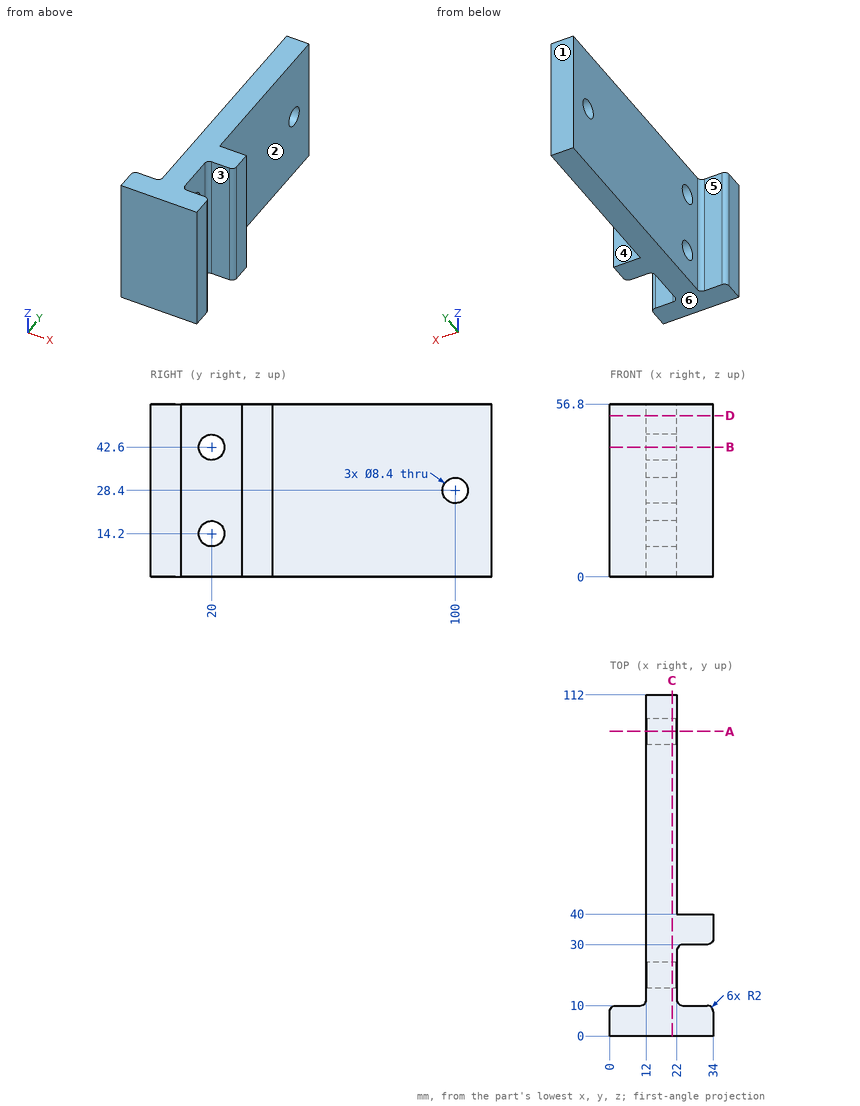
Study the drawing (mm; zero at the part's minimum x, y, z) and answer. A direction names the side the tool comes from. Round coordinates to 2 decimals unless told otherwise and drop trailing zeros. Loops run counter-clockwise (first coordinate to the right, second up) from the corner with the lowest first, then second, coordinate; pieces in that order, holes last. Notation, with made-up numbers: (-27, -36.5) -> (31, -36.5) arc R13 ccw to (31, -11.5) -> close; hole circle Ø10 at (-30, 75.5). An arc over 180 degrees is marked (long way). One line per item, written item: value.
1) For the marked faces 4, 5 and 6, determine the directions among +Z, -Z, +X, -X, +Y, -Y from which every point of the face is accessible in a straight line to the end or side of a thin tool.
Answer list:
face 4: +Z, -Z, +X, +Y
face 5: +Z, -Z, -X, +Y
face 6: -Z, +X, -X, +Y, -Y
2) The mould has two halves that part along Y. Classify the marked faces 1, 2 and 3: pulls with the +Y half, pulls with the -Y half, needs draft (parallel to the pull), parting line crosses it, or undercut.
Answer list:
face 1: pulls with the +Y half
face 2: needs draft
face 3: undercut
3) A cutting plane is placed at B-B (z = 42.6). Determine the outline of the cut face in (x, y), and give its area (3 significant figures).
Answer list:
outline: (0, 0) -> (34, 0) -> (34, 8) arc R2 ccw to (32, 10) -> (24, 10) arc R2 cw to (22, 12) -> (22, 15.8) -> (12, 15.8) -> (12, 12) arc R2 cw to (10, 10) -> (2, 10) arc R2 ccw to (0, 8) -> close; (12, 24.2) -> (22, 24.2) -> (22, 28) arc R2 cw to (24, 30) -> (32, 30) arc R2 ccw to (34, 32) -> (34, 40) -> (22, 40) -> (22, 112) -> (12, 112) -> close
area: 1,400 mm²
4) Flat-ended cylindrical pins translate along their axes: P1, Ø3, axis at y = 42, z = 49, coming from the +X side; P2, Ø9.5, axis at y = 20, z = 14.2, coming from the -X side; P3, Ø2.5, axis at x = 8, z = 26.5, coming from the +Y side. Find the tip coordinate at first contact, or state that the pin passes through.
Answer list:
P1: stops at x = 22
P2: stops at x = 12
P3: stops at y = 10
5) Consider L1, parallel to Z at x = 14, y = 20; L2, parallel to Z at x = 17, y = 100; L3, parallel to Y at x = 31, z = 33.5. Determine where each line is inside the solid, lowest interval first. Write a range as [from, to].
Answer list:
L1: z = [0, 10], [18.4, 38.4], [46.8, 56.8]
L2: z = [0, 24.2], [32.6, 56.8]
L3: y = [0, 10], [30, 40]
6) A cutting plane is placed at D-D (z = 53). Determine the outline of the cut face in (x, y).
Answer list:
outline: (0, 0) -> (34, 0) -> (34, 8) arc R2 ccw to (32, 10) -> (24, 10) arc R2 cw to (22, 12) -> (22, 28) arc R2 cw to (24, 30) -> (32, 30) arc R2 ccw to (34, 32) -> (34, 40) -> (22, 40) -> (22, 112) -> (12, 112) -> (12, 12) arc R2 cw to (10, 10) -> (2, 10) arc R2 ccw to (0, 8) -> close
7) A cutting plane is placed at C-C (x = 20.5). Determine the outline of the cut face in (y, z), and give its area (3 significant figures).
Answer list:
outline: (0, 0) -> (112, 0) -> (112, 56.8) -> (0, 56.8) -> close; hole circle Ø8.4 at (20, 14.2); hole circle Ø8.4 at (20, 42.6); hole circle Ø8.4 at (100, 28.4)
area: 6,200 mm²
8) A cutting plane is placed at A-A (y = 100). Determine the outline of the cut face in (x, z).
Answer list:
outline: (12, 0) -> (22, 0) -> (22, 24.2) -> (12, 24.2) -> close; (12, 32.6) -> (22, 32.6) -> (22, 56.8) -> (12, 56.8) -> close
